Work out the finished part from the listing and answer in its coordinate system (mm). Face numbers are marked on the shaded views. A direction names the side the tool comes from. Coordinates: 2 decimals unless noted, no trailing zeros. Loops run counter-clockwise (first coordinate to the right, second up) from the corner with the lowest first, then second, coordinate; pieces in that order, holes last. Notation, with made-up numbers: (73.25, 53) - (116.25, 53) arc R23 ccw to (116.25, 63) - close; hole circle Ø3 at (81.25, -0.75). An arc over 180 degrees is marked (long way). Write each question's results on one line, items separated by ' | '. Start each with the question number.
Item 1: A tool of negligible diameter and unlimited length cuts with its end or side. For the marked faces 1, 2 and 3, from which of +Z, -Z, +X, -X, +Y, -Y can it reach the whole face along a straight path? Write none if from no direction.
Item 2: Section A-A, the plane x = 0 is taken. Write down the section's boundary in (y, z).
Item 3: Section D-D, the plane x = -16.5 is taken. Write down the section's boundary in (y, z).
Item 4: For a pull along Y with two mould halves and no side action, classify the marked faces 4, 5 and 6 as +Y half, -Y half, draft (parallel to the pull), parting line (faces both ways), or undercut.
Item 5: Consider probe 1 along Y at (x, z) = (0, 14); probe 2 along X at (y, z) = (0.5, 9); probe 3 along Y at (x, z) = (13, 11). Determine where each line is inside the solid, lowest interval first. Write a range as [from, to].
Item 6: Section B-B, the plane z = 22 is taken. Write down the section's boundary in (x, y).
Item 7: Each of these flat-tipped pins is pushed along its axis until it touches: pin 1 Ø20 at (y, z) = (-78.5, 7.5) entering from +X; pin 2 Ø13.5 at (x, y) = (1.5, -74.5) entering from +Z; pin 3 Ø1.5 at (x, z) = (-16, 18.5) entering from +Y. Where does it stop, or does it pass through?
Item 8: Section C-C, the plane y = -32.5 is taken. Write down the section's boundary in (x, z).
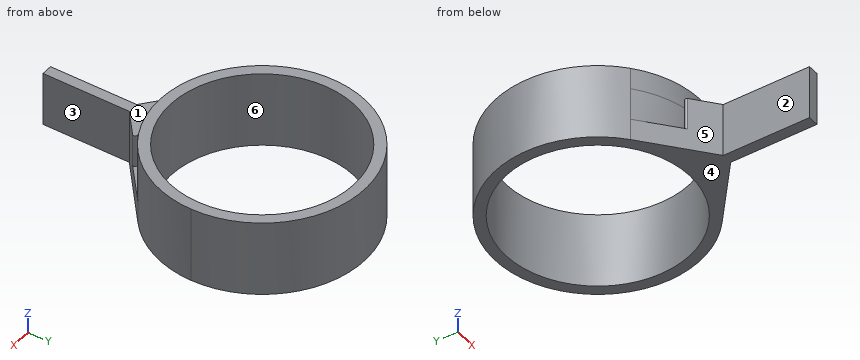
from build123d import *

# Parameters (mm, degrees)
F0_R     = 47.5
F0_R_2   = 42.5
F1_DEPTH = 35
F3_DEPTH = 25
F5_DEPTH = 25
F6_R     = 1


with BuildPart() as f1:
    # F0 (on Top) → F1 (new body)
    with BuildSketch(Plane.XY):
        Circle(F0_R)
        Circle(F0_R_2, mode=Mode.SUBTRACT)
    extrude(amount=F1_DEPTH)

    # F2 (on Top) → F3 (join)
    with BuildSketch(Plane.XY):
        Polygon((0, -47.5), (-30.5324114601, -36.3871110482), (-2.5, -59.9090971653), (-2.5, -99.9090971653), (0, -99.9090971653), (2.5, -99.9090971653), (2.5, -59.9090971653), (30.5324114601, -36.3871110482), align=None)
    extrude(amount=F3_DEPTH)

    # F4 (on face) → F5 (cut)
    with BuildSketch(Plane.XY.offset(35)):
        with BuildLine():
            ThreePointArc((30.5324114601, -36.3871110482), (0, -47.5), (-30.5324114601, -36.3871110482))
            Line((-30.5324114601, -36.3871110482), (-32.5893318111, -38.8384532661))
            ThreePointArc((-32.5893318111, -38.8384532661), (0, -50.7), (32.5893318111, -38.8384532661))
            Line((32.5893318111, -38.8384532661), (30.5324114601, -36.3871110482))
        make_face()
    extrude(amount=-F5_DEPTH, mode=Mode.SUBTRACT)

    # F6
    f6_edges = [f1.edges().sort_by_distance(p)[0] for p in [
        (16.952883, -47.781689, 17.5),
        (-16.952883, -47.781689, 17.5),
    ]]
    fillet(f6_edges, radius=F6_R)


solid = f1.part
Answer key:
1) face 1: +Z, +X, -X, -Y | face 2: +Z, -Z, -X, -Y | face 3: +Z, -Z, +X, -Y
2) outline: (-99.91, 0) - (-42.5, 0) - (-42.5, 35) - (-47.5, 35) - (-47.5, 10) - (-50.7, 10) - (-50.7, 25) - (-99.91, 25) - close; (42.5, 0) - (47.5, 0) - (47.5, 35) - (42.5, 35) - close
3) outline: (-48.16, 0) - (-39.17, 0) - (-39.17, 35) - (-44.54, 35) - (-44.54, 10) - (-48.16, 10) - close; (39.17, 0) - (44.54, 0) - (44.54, 35) - (39.17, 35) - close
4) face 4: draft | face 5: -Y half | face 6: undercut
5) probe 1: y = [-99.91, -50.7], [-47.5, -42.5], [42.5, 47.5] | probe 2: x = [-47.5, -42.5], [42.5, 47.5] | probe 3: y = [-51.1, -49.24], [-45.69, -40.46], [40.46, 45.69]
6) outline: circle Ø95 at (0, 0); (-13.22, -50.91) - (-2.5, -59.91) - (-2.5, -99.91) - (2.5, -99.91) - (2.5, -59.91) - (13.22, -50.91) arc R1 ccw to (12.34, -49.18) arc R50.7 cw to (-12.34, -49.18) arc R1 ccw to start; hole circle Ø85 at (0, 0)
7) pin 1: stops at x = 2.5 | pin 2: stops at z = 25 | pin 3: stops at y = 44.99
8) outline: (-34.64, 0) - (-27.39, 0) - (-27.39, 35) - (-34.64, 35) - close; (27.39, 0) - (34.64, 0) - (34.64, 35) - (27.39, 35) - close
